Design review of the part built by this model. Coordinates are the model's own, in mm. Coordinates: 2 decimals unless noted, no trailing zeros. Write each loop counter-clockwise with the first axis right and the second up, starting at its lowest first coordinate (ties: lowest second). Pieces come first, ordered by that corner, then holes. Notation, with made-up numbers: (-2, 43) - (27, 43) arc R27 cw to (27, 63) - close; hole circle Ø8 at (-39, 87.25). An arc over 180 degrees is marked (long way). Answer as CSV lines item,"result". Start each with the question number.
Q1. For line 1 along Z through (x, y) = (1.75, 12.7) (3 decimals); line 2 along Z through (x, y) = (12.7, 2.15) (3 decimals); line 3 along Y through (x, z) = (18.5, -161.5) (3 decimals), list the stretches that pass through material, from the lowest coordinate up. Write a range as [from, to].
Q2. We need section C-C (x = 12.7). Write out the cut boundary in (y, z) (3 decimals).
Q3. Clearance check with a flat-ended pin moving along its axis: pin 1 (5 mm diameter, centred on y = 12.7, z = -101.6, fed in from +X) (1 decimal). State where the tip first meets the part, or that it passes through.
Q4. We need section D-D (z = -110.5). Write out the cut boundary in (x, y) (3 decimals).
Q5. We need section A-A (z = -165.1). Write out the cut boundary in (x, y) (3 decimals).
Q6. We need section B-B (y = 18). Write out the cut boundary in (x, z) (3 decimals), plus the area to 3 significant figures.
Autodesk Inventor part; units mm, degrees
ref_plane "YZ Plane" through (0, 0, 0) normal (1, 0, 0) x (0, 1, 0)
ref_plane "XZ Plane" through (0, 0, 0) normal (0, 1, 0) x (-1, 0, 0)
ref_plane "XY Plane" through (0, 0, 0) normal (0, 0, 1) x (1, 0, 0)
sketch "Sketch1" plane through (0, 0, 0) normal (0, 0, 1) x (1, 0, 0)
  line L0 (0, 0) -> (25.4, 0)
  line L1 (25.4, 0) -> (25.4, 25.4)
  line L2 (25.4, 25.4) -> (0, 25.4)
  line L3 (0, 25.4) -> (0, 0)
  line L4 (3.175, 22.225) -> (22.225, 22.225)
  line L5 (22.225, 22.225) -> (22.225, 3.175)
  line L6 (22.225, 3.175) -> (3.175, 3.175)
  line L7 (3.175, 3.175) -> (3.175, 22.225)
  dimension "d0" = 25.4
  dimension "d1" = 25.4
  dimension "d2" = 3.175
extrude "Extrusion1" add sketch "Sketch1" against normal blind 203.2
sketch "Sketch2" plane through (0, 0, 0) normal (-1, 0, 0) x (0, 0, 1)
  line L0 (-203.2, 25.4) -> (-203.2, 0)
  line L1 (0, 25.4) -> (-203.2, 25.4)
  point P0 (-190.5, 12.7)
  point P1 (-165.1, 12.7)
  point P2 (-101.6, 12.7)
  dimension "d5" = 12.7
  dimension "d6" = 25.4
  dimension "d7" = 12.7
hole "Hole1" at (0, 12.7, -190.5) at (0, 12.7, -165.1) at (0, 12.7, -101.6) direction (1, 0, 0) diameter 6.35 depth 25.4 tip angle 118
sketch "Sketch3" plane through (0, 0, 0) normal (0, -1, 0) x (1, 0, 0)
  line L0 (0, 0) -> (25.4, 0)
  point P0 (12.7, -12.7)
  point P1 (12.7, -38.1)
  dimension "d15" = 25.4
  dimension "d16" = 12.7
hole "Hole2" at (12.7, 0, -12.7) at (12.7, 0, -38.1) direction (0, 1, 0) diameter 6.35 depth 25.4 tip angle 118
properties part number "towermiddle8inbrace"
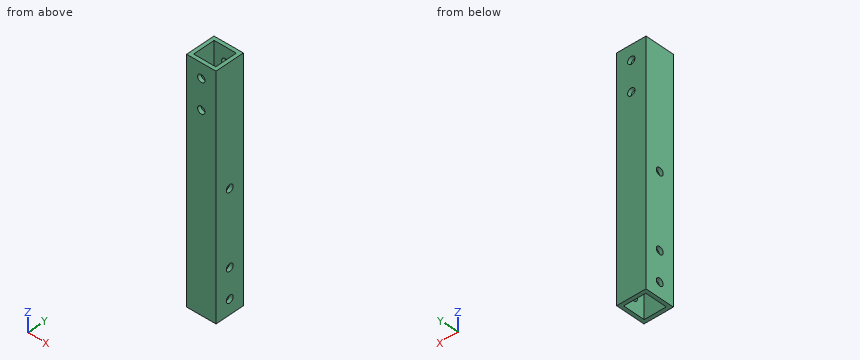
Results list:
1,line 1,"z = [-203.2, -193.675], [-187.325, -168.275], [-161.925, -104.775], [-98.425, 0]"
1,line 2,"z = [-203.2, -41.275], [-34.925, -15.875], [-9.525, 0]"
1,line 3,"y = [0, 3.175], [22.225, 25.4]"
2,outline,"(0, -203.2) - (3.175, -203.2) - (3.175, -41.275) - (0, -41.275) - close; (0, -34.925) - (3.175, -34.925) - (3.175, -15.875) - (0, -15.875) - close; (0, -9.525) - (3.175, -9.525) - (3.175, 0) - (0, 0) - close; (22.225, -203.2) - (25.4, -203.2) - (25.4, -41.275) - (22.225, -41.275) - close; (22.225, -34.925) - (25.4, -34.925) - (25.4, -15.875) - (22.225, -15.875) - close; (22.225, -9.525) - (25.4, -9.525) - (25.4, 0) - (22.225, 0) - close"
3,pin 1,"passes through"
4,outline,"(0, 0) - (25.4, 0) - (25.4, 25.4) - (0, 25.4) - close; hole (3.175, 3.175) - (22.225, 3.175) - (22.225, 22.225) - (3.175, 22.225) - close"
5,outline,"(0, 0) - (25.4, 0) - (25.4, 9.525) - (22.225, 9.525) - (22.225, 3.175) - (3.175, 3.175) - (3.175, 9.525) - (0, 9.525) - close; (0, 15.875) - (3.175, 15.875) - (3.175, 22.225) - (22.225, 22.225) - (22.225, 15.875) - (25.4, 15.875) - (25.4, 25.4) - (0, 25.4) - close"
6,outline,"(0, -203.2) - (3.175, -203.2) - (3.175, 0) - (0, 0) - close; (22.225, -203.2) - (25.4, -203.2) - (25.4, 0) - (22.225, 0) - close"
6,area,"1,290 mm2"
